Here's how the part is built. I have some questions about the finished solid (model axes, mm). Face numbers are marked on the shaded views. A direction names the side the tool comes from. Give positions to 0.01 mm unless a question says otherwise; leave off trailing zeros. Write each loop counter-clockwise with the first axis right and the second up, starting at its lowest first coordinate (ties: lowest second). Pieces come first, ordered by that corner, then holes. Notation, with made-up numbers: (71, 71.5) -> (100, 71.5) arc R9 cw to (100, 76.5) -> close; hole circle Ø7 at (70, -37.75). An arc over 180 degrees is marked (long way). Return JSON: item names as keys, results as strings.
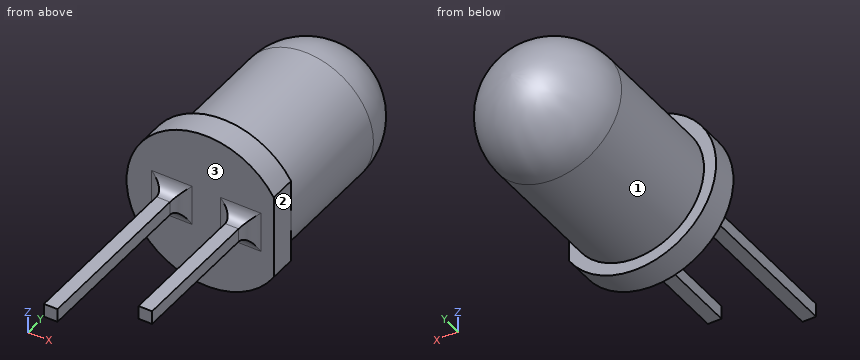
from build123d import *

# Parameters (mm, degrees)
CROQUIS1_R           = 2.95
BASE_DEPTH           = 1
CROQUIS2_R           = 2.5
CUERPO_DEL_LED_DEPTH = 7.25
CROQUIS3_W           = 0.5
CROQUIS3_H           = 0.5
PINES_DEPTH          = 7
CROQUIS4_W           = 0.5
CROQUIS4_H           = 0.5
CORTE_A_CATODO_DEPTH = 1.5
REDONDEO_A_ANODO_R   = 0.5
REDONDEO_A_CATODO_R  = 0.5
CROQUIS6_W           = 1
CROQUIS6_H           = 6
RANURA_DEPTH         = 1
PUNTA_DEL_LED_R      = 2.49


with BuildPart() as part:
    # Croquis1 → Base (new body)
    with BuildSketch(Plane(origin=(0, 0, 0), x_dir=(1, 0, 0), z_dir=(0, 1, 0))):
        Circle(CROQUIS1_R)
    extrude(amount=BASE_DEPTH)

    # Croquis2 → Cuerpo del LED (add)
    with BuildSketch(Plane(origin=(0, 1, 0), x_dir=(1, 0, 0), z_dir=(0, 1, 0))):
        Circle(CROQUIS2_R)
    extrude(amount=CUERPO_DEL_LED_DEPTH)

    # Croquis3 → Pines (add)
    with BuildSketch(Plane.XZ):
        with Locations((-1.270142923, 0)):
            Rectangle(CROQUIS3_W, CROQUIS3_H)
        with Locations((1.270172723, 0)):
            Rectangle(CROQUIS3_W, CROQUIS3_H)
    extrude(amount=PINES_DEPTH)

    # Croquis4 → Corte a Catodo (cut)
    with BuildSketch(Plane.XZ.offset(7)):
        with Locations((1.270172723, 0)):
            Rectangle(CROQUIS4_W, CROQUIS4_H)
    extrude(amount=-CORTE_A_CATODO_DEPTH, mode=Mode.SUBTRACT)

    # Redondeo a Anodo
    redondeo_a_anodo_edges = [part.edges().sort_by_distance(p)[0] for p in [
        (-1.520142923, 0, 0),
        (-1.270142923, 0, -0.25),
        (-1.020142923, 0, 0),
        (-1.270142923, 0, 0.25),
    ]]
    fillet(redondeo_a_anodo_edges, radius=REDONDEO_A_ANODO_R)

    # Redondeo a Catodo
    redondeo_a_catodo_edges = [part.edges().sort_by_distance(p)[0] for p in [
        (1.020172723, 0, 0),
        (1.270172723, 0, -0.25),
        (1.520172723, 0, 0),
        (1.270172723, 0, 0.25),
    ]]
    fillet(redondeo_a_catodo_edges, radius=REDONDEO_A_CATODO_R)

    # Croquis6 → Ranura (cut)
    with BuildSketch(Plane(origin=(0, 1, 0), x_dir=(1, 0, 0), z_dir=(0, 1, 0))):
        with Locations((3, -0.26955261)):
            Rectangle(CROQUIS6_W, CROQUIS6_H)
    extrude(amount=-RANURA_DEPTH, mode=Mode.SUBTRACT)

    # Punta del Led
    punta_del_led_edges = [part.edges().sort_by_distance(p)[0] for p in [
        (-2.5, 8.25, 0),
    ]]
    fillet(punta_del_led_edges, radius=PUNTA_DEL_LED_R)


solid = part.part
1. Which directions (+Z, -Z, +X, -X, +Y, -Y) give clear straight access to the entire face, cutting with the end or side of a thin tool? Please do the marked faces 1, 2 and 3.
Taken from the geometry:
{"face 1": "+Y", "face 2": "+Z, -Z, +X, +Y, -Y", "face 3": "-Y"}
2. For pin 1 Ø3 at (y, z) = (6.5, -0.5) entering from -X; pin 2 Ø0.6 at (x, y) = (1.5, -4) entering from -Z; pin 3 Ø1.5 at (y, z) = (-3.5, -1.5) entering from -X; pin 4 Ø3 at (x, y) = (-1, -5) entering from +Z, each with a flat end and sliding along its axis, tell me the tip position at first contact or that it passes through.
Taken from the geometry:
{"pin 1": "stops at x = -2.5", "pin 2": "stops at z = -0.25", "pin 3": "passes through", "pin 4": "stops at z = 0.25"}
3. If I drill on line 1 (Y direction, x = -2.05, z = -1.5); line 2 (Z direction, x = -0.05, y = 3.25); line 3 (Y direction, x = 0.55, z = -0.2), over which ranges is the centre line in solid material (lowest first)? Write a range as [from, to].
Taken from the geometry:
{"line 1": "y = [0, 1]", "line 2": "z = [-2.5, 2.5]", "line 3": "y = [0, 8.18]"}
4. Suppose I cut it at B-B, the plane y = 3. List the corners of the cut face in (x, z) for me, and give its area (3 significant figures).
Taken from the geometry:
{"outline": "circle Ø5 at (0, 0)", "area": "19.6 mm²"}
5. Suppose I cut it at A-A, the plane y = -2.5. List the corners of the cut face in (x, z) for me, and give its area (3 significant figures).
Taken from the geometry:
{"outline": "(-1.52, -0.25) -> (-1.02, -0.25) -> (-1.02, 0.25) -> (-1.52, 0.25) -> close; (1.02, -0.25) -> (1.52, -0.25) -> (1.52, 0.25) -> (1.02, 0.25) -> close", "area": "0.500 mm²"}
